```python
from build123d import *

# Parameters (mm, degrees)
SKETCH1_W           = 177.8
SKETCH1_H           = 203.2
BOSS_EXTRUDE2_DEPTH = 76.2
SKETCH3_W           = 127
SKETCH3_H           = 88.9
CUT_EXTRUDE1_DEPTH  = 76.2
SKETCH4_R           = 19.05
CUT_EXTRUDE3_DEPTH  = 199.898


with BuildPart() as part:
    # Sketch1 → Boss-Extrude2 (new body)
    with BuildSketch(Plane.XY):
        with Locations((88.9, 101.6)):
            Rectangle(SKETCH1_W, SKETCH1_H)
    extrude(amount=BOSS_EXTRUDE2_DEPTH)

    # Sketch3 → Cut-Extrude1 (cut)
    with BuildSketch(Plane.XY.offset(76.2)):
        with Locations((88.9, 158.75)):
            Rectangle(SKETCH3_W, SKETCH3_H)
        with Locations((88.9, 44.45)):
            Rectangle(SKETCH3_W, SKETCH3_H)
    extrude(amount=-CUT_EXTRUDE1_DEPTH, mode=Mode.SUBTRACT)

    # Sketch4 → Cut-Extrude3 (cut)
    with BuildSketch(Plane.ZY):
        with Locations((38.1, 171.45)):
            Circle(SKETCH4_R)
        with Locations((38.1, 31.75)):
            Circle(SKETCH4_R)
    extrude(amount=-CUT_EXTRUDE3_DEPTH, mode=Mode.SUBTRACT)


solid = part.part
```
CAD build for the part. Positions are in the model's coordinates, mm. A direction names the side the tool comes from. Round coordinates to 2 decimals unless told otherwise and drop trailing zeros. Order: outer loops, then holes, each group sorted by start corner. A loop starts at its lowest first (then second) coordinate and runs counter-clockwise, first axis right, second up. Notation, with made-up numbers: (29, 28) - (48, 28) arc R12 ccw to (48, 50) - close; hole circle Ø7 at (-3, -21.75). An arc over 180 degrees is marked (long way). Answer in a Markdown table with one row per item. Add a question column.
(1) Mould opens along Z. For faces 1 (the face through (164.922, 50.638, 35.62)), 2 (the face through (88, 110, 0)), 3 (the face through (88, 110, 76.2)), 4 (the face through (13, 203.2, 38)) say: +Z half, -Z half, draft (parallel to the pull), parting line (faces both ways), or undercut.
(2) Band-saw the part on A-A on y = 149. List the corners of the cut face in (x, z), and give its area (3 significant figures).
(3) Probe L1, parallel to Y at x = 168, z = 38; L2, parallel to Y at x = 22, z = 39.5; L3, parallel to X at y = 46.5, z = 69. List the from-to ranges inside material, lowest first. Write a range as [from, to].
(4) Band-saw the part on B-B on z = 38.1. List the corners of the cut face in (x, y).
(5) Band-saw the part on D-D on x = 126.5. List the corners of the cut face in (y, z).
(6) Drop a flat-ended pin along its axis: pin 1 Ø3 at (x, z) = (62.5, 35) entering from +Y. Give the stop position or say it passes through.
(7) 3-axis set-ups, long thin cutter, end or side, ignore diameter. For faces 5 (the face through (165, 203.2, 38)), 6 (the face through (25.4, 148, 39)), 7 (the face through (25.4, 54, 39)): which of +Z, -Z, +X, -X, +Y, -Y reach the whole face in a straight line?
(8) Band-saw the part on C-C on y = 171.45. List the corners of the cut face in (x, z), and give its area (3 significant figures).
Data:
| question | item | result |
|---|---|---|
| 1 | face 1 | undercut |
| 1 | face 2 | -Z half |
| 1 | face 3 | +Z half |
| 1 | face 4 | draft |
| 2 | outline | (0, 0) - (25.4, 0) - (25.4, 76.2) - (0, 76.2) - close; (152.4, 0) - (177.8, 0) - (177.8, 76.2) - (152.4, 76.2) - close |
| 2 | area | 3,870 mm^2 |
| 3 | L1 | y = [0, 12.7], [50.8, 152.4], [190.5, 203.2] |
| 3 | L2 | y = [0, 12.75], [50.75, 152.45], [190.45, 203.2] |
| 3 | L3 | x = [0, 25.4], [152.4, 177.8] |
| 4 | outline | (0, 0) - (25.4, 0) - (25.4, 12.7) - (0, 12.7) - close; (0, 50.8) - (25.4, 50.8) - (25.4, 88.9) - (152.4, 88.9) - (152.4, 50.8) - (177.8, 50.8) - (177.8, 152.4) - (152.4, 152.4) - (152.4, 114.3) - (25.4, 114.3) - (25.4, 152.4) - (0, 152.4) - close; (0, 190.5) - (25.4, 190.5) - (25.4, 203.2) - (0, 203.2) - close; (152.4, 0) - (177.8, 0) - (177.8, 12.7) - (152.4, 12.7) - close; (152.4, 190.5) - (177.8, 190.5) - (177.8, 203.2) - (152.4, 203.2) - close |
| 5 | outline | (88.9, 0) - (114.3, 0) - (114.3, 76.2) - (88.9, 76.2) - close |
| 6 | pin 1 | stops at y = 114.3 |
| 7 | face 5 | +Z, -Z, +X, -X, +Y |
| 7 | face 6 | +Z, -Z, +Y |
| 7 | face 7 | +Z, -Z, -Y |
| 8 | outline | (0, 0) - (25.4, 0) - (25.4, 19.05) - (0, 19.05) - close; (0, 57.15) - (25.4, 57.15) - (25.4, 76.2) - (0, 76.2) - close; (152.4, 0) - (177.8, 0) - (177.8, 19.05) - (152.4, 19.05) - close; (152.4, 57.15) - (177.8, 57.15) - (177.8, 76.2) - (152.4, 76.2) - close |
| 8 | area | 1,940 mm^2 |
